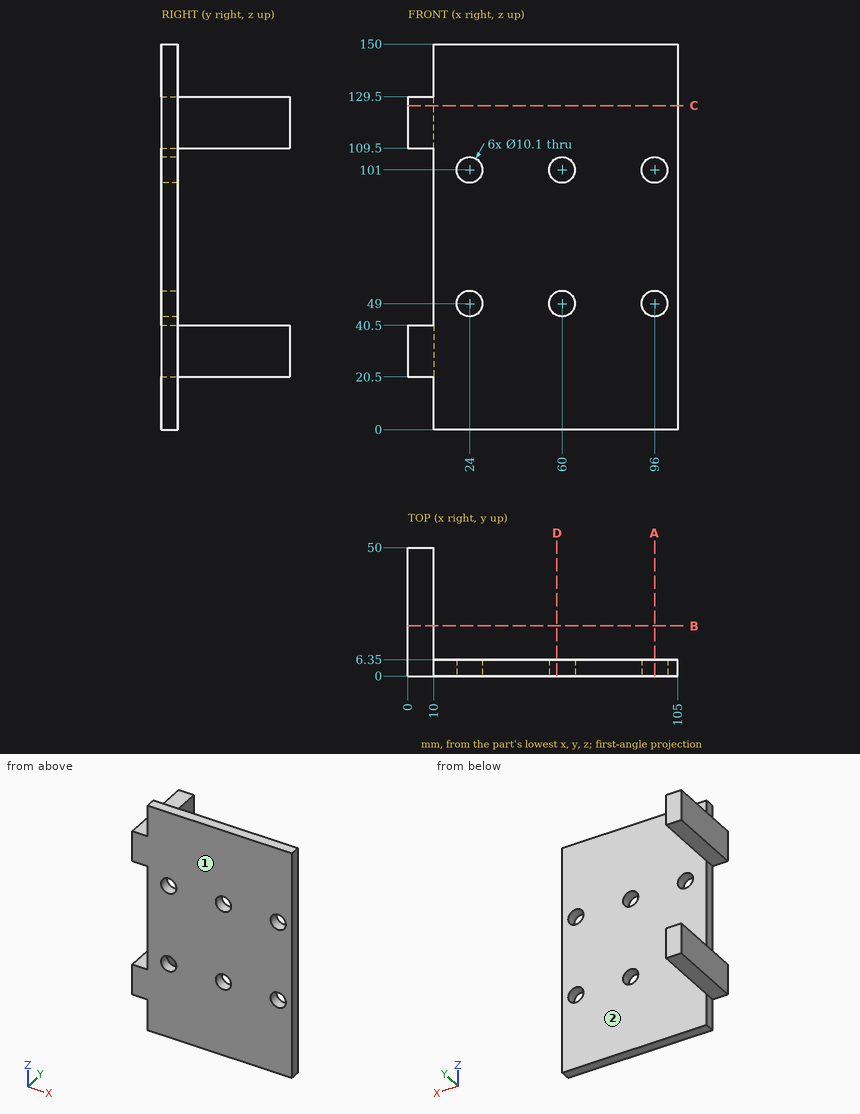
Design review of the part shown in the three views and the two pictorial views. Dimensions are in mm from the part's minimum x, y and z. A direction names the side the tool comes from. Round coordinates to 2 decimals unless told otherwise and drop trailing zeros. Loops run counter-clockwise (first coordinate to the right, second up) from the corner with the lowest first, then second, coordinate; pieces in that order, holes last. Notation, with made-up numbers: (82.25, 86.5) - (111.25, 86.5) arc R27 cw to (111.25, 116.5) - close; hole circle Ø4 at (45.25, -13.5). An arc over 180 degrees is marked (long way). Use one line per item in the form item = value.
1) Wall thickness on probe 1 along X at (y, z) = (4, 49); probe 2 along Z at (x, y) = (8, 21); probe 3 along X at (y, z) = (45, 23): over which ranges is each line inside the solid? List them lowest first.
Solutions:
probe_1 = 10 to 18.95, 29.05 to 54.95, 65.05 to 90.95, 101.05 to 105
probe_2 = 20.5 to 40.5, 109.5 to 129.5
probe_3 = 0 to 10
2) Clearance check with flat-ended pins moving along their axes: P1, Ø8, axis at x = 11, z = 131, coming from the -Y side; P2, Ø11, axis at x = 3.5, y = 31, coming from the +Z side; P3, Ø5, axis at y = 3.5, z = 73.5, coming from the -X side; P4, Ø5, axis at x = 60, z = 26, coming from the +Y side. State where each tip first meets the part, or that it passes through.
Solutions:
P1 = 0
P2 = 129.5
P3 = 10
P4 = 6.35
3) We need section C-C on z = 126. Write out the cut boundary in (x, y), then the cut area to 3 significant figures.
Solutions:
outline = (0, 0) - (105, 0) - (105, 6.35) - (10, 6.35) - (10, 50) - (0, 50) - close
area = 1,100 mm2
4) We need section B-B on y = 19.5. Write out the cut boundary in (x, z), then the cut area to 3 significant figures.
Solutions:
outline = (0, 20.5) - (10, 20.5) - (10, 40.5) - (0, 40.5) - close; (0, 109.5) - (10, 109.5) - (10, 129.5) - (0, 129.5) - close
area = 400 mm2
5) Tool access review of the marked faces 1 and 2: name each direction out of +Z, -Z, +X, -X, +Y, -Y from which nothing blocks a thin tool from reaching the whole face with its end or side.
Solutions:
face_1 = +Z, -Z, +X, -X, -Y
face_2 = +Z, -Z, +X, +Y
6) We need section D-D on x = 58. Write out the cut boundary in (y, z).
Solutions:
outline = (0, 0) - (6.35, 0) - (6.35, 44.36) - (0, 44.36) - close; (0, 53.64) - (6.35, 53.64) - (6.35, 96.36) - (0, 96.36) - close; (0, 105.64) - (6.35, 105.64) - (6.35, 150) - (0, 150) - close
7) We need section A-A on x = 96. Write out the cut boundary in (y, z), then the cut area to 3 significant figures.
Solutions:
outline = (0, 0) - (6.35, 0) - (6.35, 43.95) - (0, 43.95) - close; (0, 54.05) - (6.35, 54.05) - (6.35, 95.95) - (0, 95.95) - close; (0, 106.05) - (6.35, 106.05) - (6.35, 150) - (0, 150) - close
area = 824 mm2
